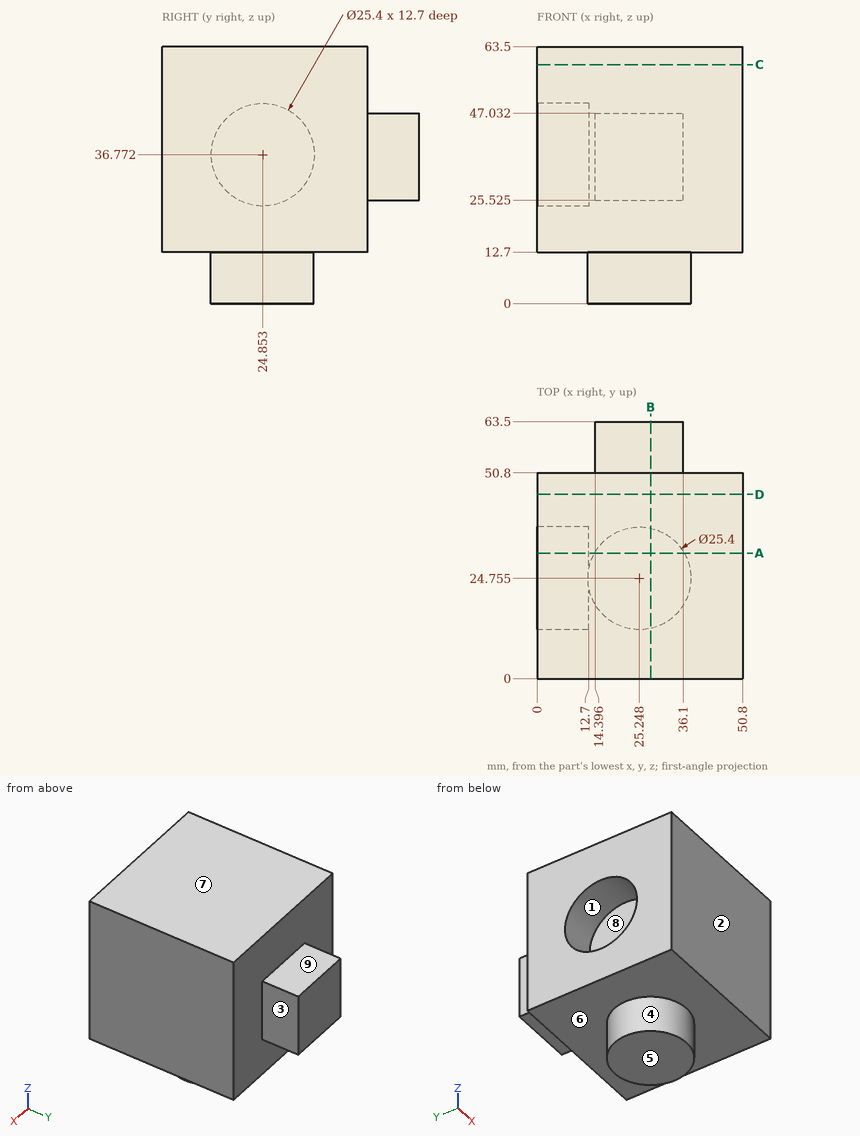
Print and shaded views of the part. All mm, measured from the part's lowest x, y and z. A direction names the side the tool comes from. Give positions to 0.01 mm unless a question says otherwise; leave off trailing zeros. Loops run counter-clockwise (first coordinate to the right, second up) from the corner with the lowest first, then second, coordinate; pieces in that order, holes last. Notation, with made-up numbers: (53.25, -9.75) -> (69.25, -9.75) arc R12 cw to (69.25, -0.75) -> close; hole circle Ø10 at (2, 22). An arc over 180 degrees is marked (long way). One line per question, with ' | ' between items. Start each with the question number.
1) Cut at C-C (z = 59). Give the cut face in (x, y).
2) Two-plate mould, pull along Y, no slides. Class the marked faces 1, 2, 3 and 4: released by +Y, released by -Y, zero draft, split by the parting line, or undercut.
3) Cut at A-A (y = 31). Give the cut face in (x, z) (1 decimal), plus the area to 3 significant figures.
4) Cut at D-D (y = 45.5). Give the cut face in (x, z), plus the area to 3 significant figures.
5) Pin check, flat tips, straight feed: pin 1 (10 mm diameter, centred on x = 22, y = 57.5, fed in from -Z) (1 decimal); pin 2 (4 mm diameter, centred on y = 55.5, z = 31.5, fed in from +X); pin 3 (14 mm diameter, centred on y = 59.5, z = 41, fed in from -X). Stop position of each tip, or through.
6) Probe L1, parallel to Y at x = 43, z = 57; L2, parallel to X at y = 34, z = 32.5; L3, parallel to Z at x = 38, y = 8. List the from-to ranges inside material, lowest first.
7) 3-axis set-ups, long thin cutter, end or side, ignore diameter. For the marked faces 5, 6, 7, 8 and 9: which of +Z, -Z, +X, -X, +Y, -Y reach the whole face in a straight line?
8) Cut at B-B (x = 28). Give the cut face in (y, z) (1 decimal).
Return value:
1) outline: (0, 0) -> (50.8, 0) -> (50.8, 50.8) -> (0, 50.8) -> close
2) face 1: undercut | face 2: released by -Y | face 3: zero draft | face 4: split by the parting line
3) outline: (0, 12.7) -> (14.2, 12.7) -> (14.2, 0) -> (36.3, 0) -> (36.3, 12.7) -> (50.8, 12.7) -> (50.8, 63.5) -> (0, 63.5) -> (0, 47.9) -> (12.7, 47.9) -> (12.7, 25.7) -> (0, 25.7) -> close | area: 2,580 mm^2
4) outline: (0, 12.7) -> (50.8, 12.7) -> (50.8, 63.5) -> (0, 63.5) -> close | area: 2,580 mm^2
5) pin 1: z = 25.5 | pin 2: x = 36.1 | pin 3: x = 14.4
6) L1: 0 to 50.8 | L2: 12.7 to 50.8 | L3: 12.7 to 63.5
7) face 5: -Z, +X, -X, +Y, -Y | face 6: -Z | face 7: +Z, +X, -X, +Y, -Y | face 8: -X | face 9: +Z, +X, -X, +Y
8) outline: (0, 12.7) -> (12.4, 12.7) -> (12.4, 0) -> (37.2, 0) -> (37.2, 12.7) -> (50.8, 12.7) -> (50.8, 25.5) -> (63.5, 25.5) -> (63.5, 47) -> (50.8, 47) -> (50.8, 63.5) -> (0, 63.5) -> close
